Design review of the part shown in the three views and the two pictorial views. Dimensions are in mm from the part's minimum x, y and z. A direction names the side the tool comes from. Round coordinates to 2 decimals unless told otherwise and drop trailing zeros. Order: outer loops, then holes, each group sorted by start corner. A loop starts at its lowest first (then second) coordinate and runs counter-clockwise, first axis right, second up. Notation, with made-up numbers: M -39,89 L 18,89 A30 ccw 18,111 Z; hole C -38.75,72 d5. An arc over 180 degrees is marked long. Write item = value, one per line. Start each with the question number.
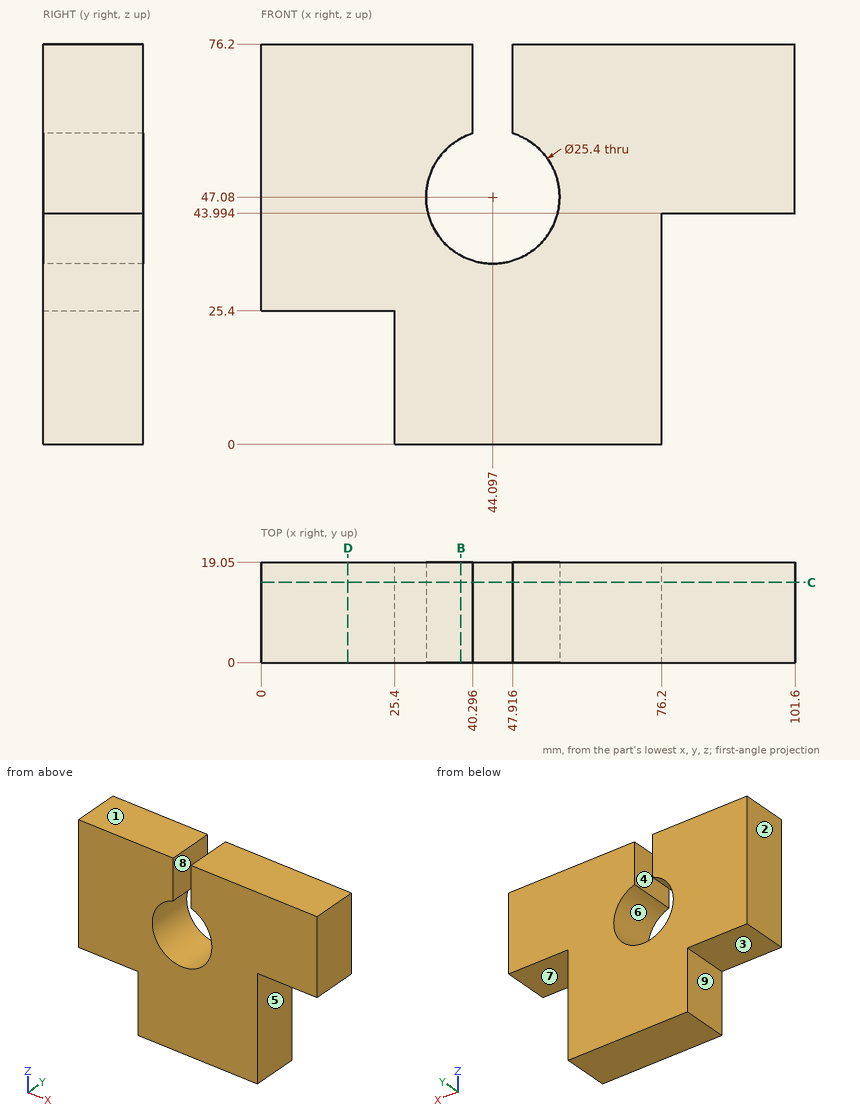
(1) We need section C-C, the plane y = 15.25. Write out the cut boundary in (x, z) (1 decimal), then the cut area to 3 significant figures.
(2) We need section B-B, the plane x = 38. Write out the cut boundary in (y, z), then the cut area to 3 significant figures.
(3) Insertion check: pin 1 (10 mm diameter, centred on y = 16.5, z = 39.5, fed in from +X); pin 2 (5.5 mm diameter, centred on y = 5.5, z = 12, fed in from -X); pin 3 (12 mm diameter, centred on x = 86, z = 18.5, fed in from -Y); pin 4 (6 mm diameter, centred on y = 9, z = 37.5, fed in from +X). Each pin has a flat end and moves straight along its axis. Give the tip position at first contact, or say it passes through.
(4) We need section D-D, the plane x = 16.5. Write out the cut boundary in (y, z).
(5) For the marked faces 1, 2, 3, 4 and 5, list the 3-axis set-ups (+Z, -Z, +X, -X, +Y, -Y) from which the entire face can be reached by the end or side of a thin tool; tool diameter is ignored.
(6) For line 1 along X through (y, z) = (13.25, 66) (1 decimal); line 2 along X through (y, z) = (13.25, 18.5); line 3 along Z through (x, y) = (96.5, 1.5), list the stretches that pass through material, from the lowest coordinate up.
(7) Draft analysis for pull direction X (two halves, no side actions). For the marked faces 6, 7, 8 and 9, state which applies: released by +X, released by -X, zero draft, split by the parting line, or undercut.
Values:
q1.outline = M 0,25.4 L 25.4,25.4 L 25.4,0 L 76.2,0 L 76.2,44 L 101.6,44 L 101.6,76.2 L 47.9,76.2 L 47.9,59.2 A12.7 cw long 40.3,59.2 L 40.3,76.2 L 0,76.2 Z
q1.area = 5,350 mm²
q2.outline = M 0,0 L 19.05,0 L 19.05,35.94 L 0,35.94 Z; M 0,58.22 L 19.05,58.22 L 19.05,76.2 L 0,76.2 Z
q2.area = 1,030 mm²
q3.pin_1 = 101.6
q3.pin_2 = 25.4
q3.pin_3 = through
q3.pin_4 = 76.2
q4.outline = M 0,25.4 L 19.05,25.4 L 19.05,76.2 L 0,76.2 Z
q5.face_1 = +Z, +X, -X, +Y, -Y
q5.face_2 = +Z, -Z, -X, +Y, -Y
q5.face_3 = -Z, -X, +Y, -Y
q5.face_4 = +Z, +Y, -Y
q5.face_5 = -Z, +X, +Y, -Y
q6.line_1 = 0 to 40.3, 47.9 to 101.6
q6.line_2 = 25.4 to 76.2
q6.line_3 = 43.99 to 76.2
q7.face_6 = undercut
q7.face_7 = zero draft
q7.face_8 = undercut
q7.face_9 = released by -X
